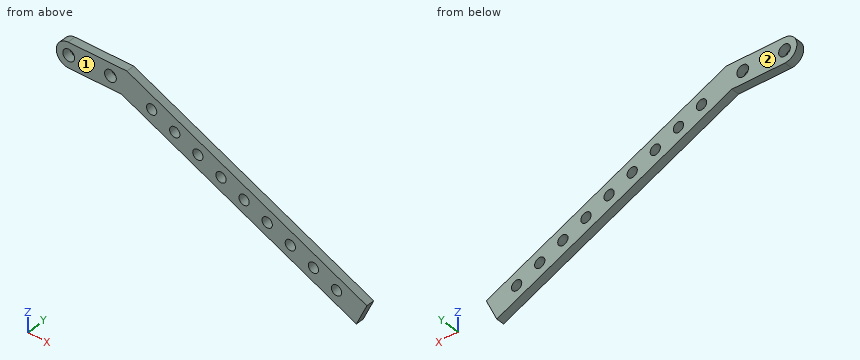
Autodesk Inventor part; units mm, degrees
ref_plane "YZ Plane" through (0, 0, 0) normal (1, 0, 0) x (0, 1, 0)
ref_plane "XZ Plane" through (0, 0, 0) normal (0, 1, 0) x (-1, 0, 0)
ref_plane "XY Plane" through (0, 0, 0) normal (0, 0, 1) x (1, 0, 0)
sketch "Sketch1" plane through (0, 0, 0) normal (0, 1, 0) x (-1, 0, 0)
  line L0 (0, 0) -> (22.5338, 0)
  line L1 (22.5244, -9.525) -> (-0.0054, -9.525)
  line L2 (-0.0054, -9.525) -> (0, 0)
  arc A0 (22.5244, -9.525) -> (22.5338, 0) centre (22.3099, -4.7623) ccw
  line L3 (0, 0) -> (-92.0441, -42.9209)
  line L4 (0, 0) -> (101.5594, 0) construction
  line L5 (-92.0441, -42.9209) -> (-88.0186, -51.5534)
  line L6 (0, 0) -> (4.0254, -8.6326)
  line L7 (4.0254, -8.6326) -> (-88.0186, -51.5534)
  circle A1 centre (22.3099, -4.7623) radius 2.2479
  line L8 (22.3099, -4.7623) -> (6.3079, -4.7623) construction
  circle A2 centre (6.3079, -4.7623) radius 2.2479
  line L9 (2.0127, -4.3163) -> (-9.4974, -9.6835) construction
  circle A3 centre (-9.4974, -9.6835) radius 1.9685
  line L10 (2.0127, -4.3163) -> (-90.0313, -47.2371) construction
  circle A4 centre (-18.3602, -13.8163) radius 1.9685
  circle A5 centre (-27.223, -17.9491) radius 1.9685
  circle A6 centre (-36.0857, -22.0819) radius 1.9685
  circle A7 centre (-44.9485, -26.2147) radius 1.9685
  circle A8 centre (-53.8113, -30.3475) radius 1.9685
  circle A9 centre (-62.6741, -34.4802) radius 1.9685
  circle A10 centre (-71.5369, -38.613) radius 1.9685
  circle A11 centre (-80.3997, -42.7458) radius 1.9685
  line L11 (22.3099, -4.7623) -> (6.1972, -4.7623) construction
  line L12 (6.1972, -4.7623) -> (6.1972, 11.2397) construction
  line L13 (6.1972, 11.2397) -> (22.3099, 11.2397) construction
  line L14 (22.3099, 11.2397) -> (22.3099, -4.7623) construction
  line L15 (14.2536, 11.2397) -> (14.2536, -4.7623) construction
  line L16 (22.3099, 3.2387) -> (6.1972, 3.2387) construction
  circle A12 centre (14.2536, 3.2387) radius 1.27 construction
  dimension "d0" = 22.5298
  dimension "d1" = 9.525
  dimension "d2" = 4.7675
  dimension "d4" = 155
  dimension "d7" = 9.525
  dimension "d8" = 9.525
  dimension "d9" = 4.4958
  dimension "d10" = 16.002
  dimension "d11" = 4.4958
  dimension "d12" = 12.7
  dimension "d13" = 3.937
  dimension "d14" = 4.7625
  dimension "d15" = 3.937
  dimension "d16" = 9.779
  dimension "d17" = 3.937
  dimension "d18" = 9.779
  dimension "d19" = 3.937
  dimension "d20" = 9.779
  dimension "d21" = 3.937
  dimension "d22" = 9.779
  dimension "d23" = 3.937
  dimension "d24" = 9.779
  dimension "d25" = 3.937
  dimension "d26" = 9.779
  dimension "d27" = 3.937
  dimension "d28" = 9.779
  dimension "d29" = 3.937
  dimension "d30" = 9.779
  dimension "d31" = 16.002
  dimension "d32" = 2.54
  dimension "d33" = 115.8874
extrude "Extrusion1" add sketch "Sketch1" along normal blind 3.175
properties part number "CollectorArm155"
Geometry check sheet. Reference: the model listing, model coordinates, mm. Face numbers are marked on the shaded views. Give positions to 0.01 mm unless a question says otherwise; leave off trailing zeros. Write each loop counter-clockwise with the first axis right and the second up, starting at its lowest first coordinate (ties: lowest second). Pieces come first, ordered by that corner, then holes. Notation, with made-up numbers: (7.25, 54.5) - (51.25, 54.5) arc R20 ccw to (51.25, 79.5) - close; hole circle Ø11 at (-6.5, 0). An arc over 180 degrees is marked (long way). Put each result on its own line as item: value.
1. Draft check along Y on the marked faces 1 and 2. Enter one of: +Y half, -Y half, draft (parallel to the pull), parting line (faces both ways), or undercut.
Ans:
face 1: -Y half
face 2: +Y half
2. Sectioned sample at C-C, the plane x = 17.5. Enter the section's corners in (y, z) (3 decimals), plus the area to 3 significant figures.
Ans:
outline: (0, -18.67) - (3.175, -18.67) - (3.175, -15.587) - (0, -15.587) - close; (0, -12.046) - (3.175, -12.046) - (3.175, -8.16) - (0, -8.16) - close
area: 22.1 mm²
3. Thickness scan on line 1 (X direction, y = 2.9, z = -3); line 2 (X direction, y = 0.95, z = -37.5); line 3 (Z direction, x = -18, y = 0.5) (3 decimals). Record the ranges inside material, lowest first.
Ans:
line 1: x = -26.74 to -23.71, -20.91 to -7.7, -4.91 to 6.43
line 2: x = 57.88 to 69.91, 73.16 to 80.42
line 3: z = -9.525 to 0
4. Go/stop test with flat-tipped pins: pin 1 (5 mm diameter, centred on x = 80.4, z = -42.75, fed in from -Y); pin 2 (1 mm diameter, centred on x = 39.5, y = 2, fed in from +Z). Record where each tip stops, or that it passes through.
Ans:
pin 1: stops at y = 0
pin 2: stops at z = -18.19
5. Sectioned sample at B-B, the plane y = 1.35. Give the number of separate pieces and of enclosed holes in the cut face, plus the area to 3 significant figures.
Ans:
separate pieces: 1
enclosed holes: 11
area: 1,050 mm²
6. Sectioned sample at A-A, the plane x = 35.5. Enter the section's corners in (y, z) (3 decimals), plus the area to 3 significant figures.
Ans:
outline: (0, -27.064) - (3.175, -27.064) - (3.175, -23.961) - (0, -23.961) - close; (0, -20.203) - (3.175, -20.203) - (3.175, -16.554) - (0, -16.554) - close
area: 21.4 mm²
